Check sheet for the drawn part. Datum: minimum x, y, z corner. Units: mm. Give positions to 0.01 mm unless a question says otherwise; leave off trailing zeros. Write each loop counter-clockwise with the first axis right and the second up, starting at its lowest first coordinate (ties: lowest second). Pieces come first, ordered by that corner, then holes. Notation, with made-up numbers: (-24, -38.5) - (-5, -38.5) arc R12 cw to (-5, -17.5) - close; hole circle Ø11 at (-10.5, 7.25). An arc over 180 degrees is marked (long way). One line per question, with ' | ' between items. Start each with the question number.
Q1. Section check C-C on y = 54.5. Record the boundary of the cut face in (x, z), and give its area (3 significant figures).
Q2. Section check B-B on z = 2.5. Record the boundary of the cut face in (x, y).
Q3. Thickness scan on L1, parallel to Z at x = 2.7, y = 54; L2, parallel to Y at x = 0.3, z = 2. Record the ranges inside material, lowest first. Write a range as [from, to].
Q4. Section check A-A on x = 1.35. Record the boundary of the cut face in (y, z), and give its area (3 significant figures).
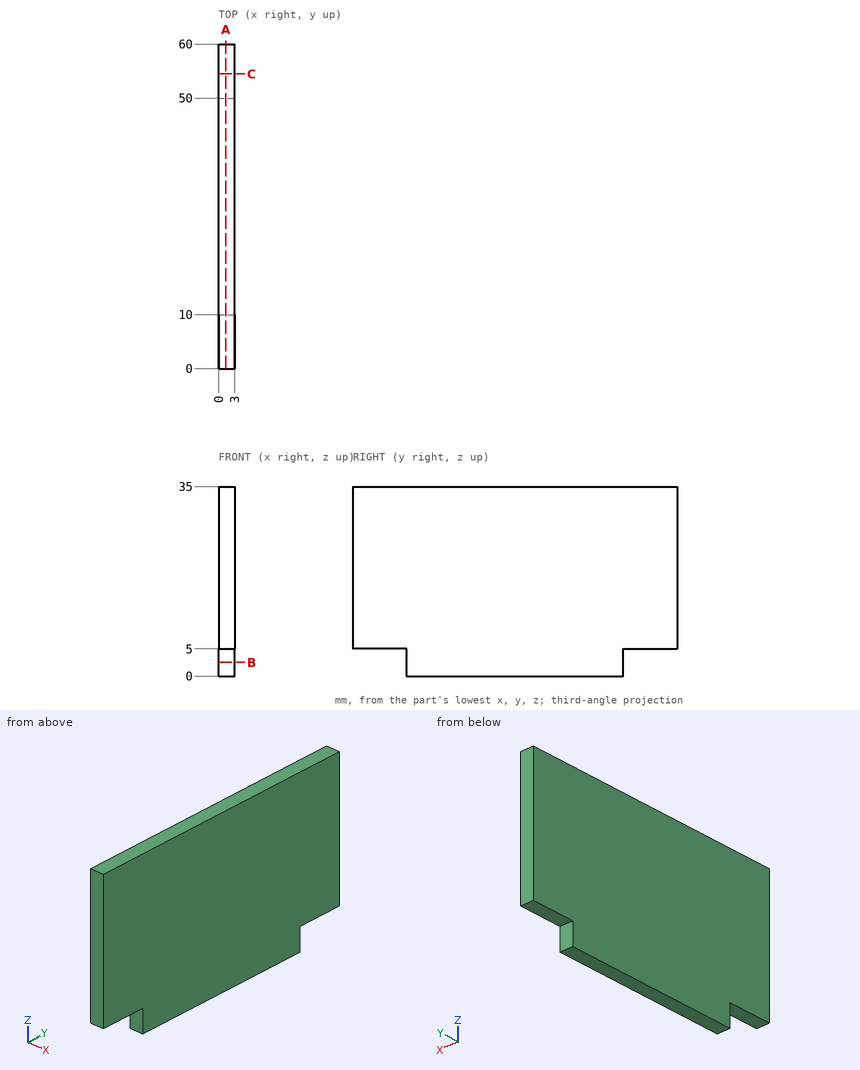
Working result:
1) outline: (0, 5) - (3, 5) - (3, 35) - (0, 35) - close | area: 90.0 mm2
2) outline: (0, 10) - (3, 10) - (3, 50) - (0, 50) - close
3) L1: z = [5, 35] | L2: y = [10, 50]
4) outline: (0, 5) - (10, 5) - (10, 0) - (50, 0) - (50, 5) - (60, 5) - (60, 35) - (0, 35) - close | area: 2,000 mm2
